Part model, mm, in its own coordinate system. Give positions to 0.01 mm unless a question says otherwise; leave off trailing zeros. Order: outer loops, then holes, each group sorted by start corner. A loop starts at its lowest first (then second) coordinate and runs counter-clockwise, first axis right, second up. Notation, with made-up numbers: M 22,89 L 40,89 A22 cw 40,102 Z; hole C 15,31 d1. An arc over 180 degrees is marked long. Answer as a JSON object with one key per item and string values.
from build123d import *

# Parameters (mm, degrees)
BOSS_EXTRUDE1_DEPTH = 20.32
SKETCH3_R           = 2.6
CUT_EXTRUDE1_DEPTH  = 10.16
CIRPATTERN1_COUNT   = 4


with BuildPart() as part:
    # Sketch2 → Boss-Extrude1 (new body)
    with BuildSketch(Plane(origin=(0, 0, 0), x_dir=(1, 0, 0), z_dir=(0, 1, 0))):
        Polygon((-9.999999999999998, 10), (10.000000000000002, 10), (10.000000000000005, -10), (-9.999999999999995, -10), align=None)
    extrude(amount=BOSS_EXTRUDE1_DEPTH)

    # Sketch3 → Cut-Extrude1 (cut)
    with BuildSketch(Plane.XY.offset(10)):
        with Locations((8.7e-16, 10.16)):
            Circle(SKETCH3_R)
    cut_extrude1 = extrude(amount=-CUT_EXTRUDE1_DEPTH, mode=Mode.SUBTRACT)

    # CirPattern1: Cut-Extrude1 ×4 about axis
    cirpattern1_axis = Axis((1.73e-15, 20.32, 0), (-9e-17, -1, 0))
    for i in range(1, CIRPATTERN1_COUNT):
        add(cut_extrude1.rotate(cirpattern1_axis, i * 360 / CIRPATTERN1_COUNT), mode=Mode.SUBTRACT)


solid = part.part
1. Cut at A-A on y = 10.16. Give the cut face in (x, z).
Worked answers:
{"outline": "M -10,-10 L -2.6,-10 L -2.6,-2.6 L -10,-2.6 Z; M -10,2.6 L -2.6,2.6 L -2.6,10 L -10,10 Z; M 2.6,-10 L 10,-10 L 10,-2.6 L 2.6,-2.6 Z; M 2.6,2.6 L 10,2.6 L 10,10 L 2.6,10 Z"}
2. Two-plate mould, pull along X, no slides. Class faces 1 (the cylindrical face through (1.4, 7.97, 6.04)), 2 (the flat face through (10, 8, -2)), 3 (the flat face through (0, 0, 0)): +X half, -X half, draft (parallel to the pull), parting line (faces both ways), or undercut.
Worked answers:
{"face 1": "undercut", "face 2": "+X half", "face 3": "draft"}
3. Cut at D-D on x = -1.25. Give the cut face in (y, z), plus the area to 3 significant figures.
Worked answers:
{"outline": "M 0,-10 L 7.88,-10 L 7.88,-1.25 A2.6 cw 7.88,1.25 L 7.88,10 L 0,10 Z; M 12.44,-10 L 20.32,-10 L 20.32,10 L 12.44,10 L 12.44,1.25 A2.6 cw 12.44,-1.25 Z", "area": "314 mm^2"}
4. Cut at C-C on z = -7.25. Give the cut face in (x, y), plus the area to 3 significant figures.
Worked answers:
{"outline": "M -10,0 L 10,0 L 10,20.32 L -10,20.32 Z; hole C 0,10.16 d5.2", "area": "385 mm^2"}
5. Probe line 1 along Y through (x, z) = (0, 7.25); line 2 along X through (y, z) = (10.16, -3.75). List the from-to ranges inside material, lowest first.
Worked answers:
{"line 1": "y = 0 to 7.56, 12.76 to 20.32", "line 2": "x = -10 to -2.6, 2.6 to 10"}
6. Cut at B-B on x = -7.75. Give the cut face in (y, z).
Worked answers:
{"outline": "M 0,-10 L 20.32,-10 L 20.32,10 L 0,10 Z; hole C 10.16,0 d5.2"}
